Study the drawing (mm; zero at the part's minimum x, y, z) and answer. A direction names the side the tool comes from. Coordinates: 2 decimals unless noted, no trailing zeros. Order: outer loops, then holes, each group sorted by start corner. A loop starts at its lowest first (then second) coordinate and runs counter-clockwise, first axis right, second up. Notation, with made-up numbers: M 7.25,83 L 25.25,83 A36 ccw 25.25,119 Z; hole C 25.25,-2.75 d10. An arc over 180 degrees is marked long. Use a Markdown table: item, result. Add a question column.
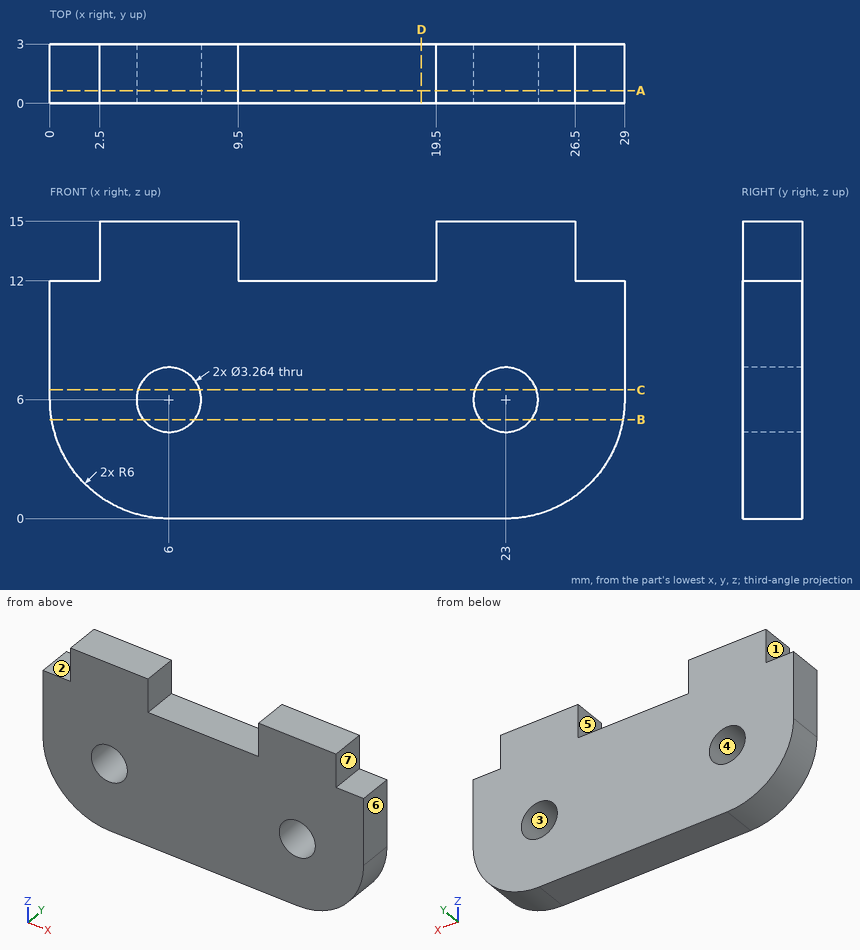
(1) A cutting plane is placed at B-B on z = 5. Write down the section's boundary in (x, y).
(2) The mould has two halves that part along X. Classify the marked faces 1, 2, 3 and 4: pulls with the +X half, pulls with the -X half, needs draft (parallel to the pull), parting line crosses it, or undercut.
(3) A cutting plane is placed at D-D on x = 18.75. Write down the section's boundary in (y, z).
(4) Straight lines are drawn through the part: line 1 (X direction, y = 2.2, z = 6); line 2 (Z direction, x = 23, y = 0.7); line 3 (X direction, y = 2.6, z = 6.75). For each, find the intervals that lie inside material, in ascending order.
(5) A cutting plane is placed at C-C on z = 6.5. Write down the section's boundary in (x, y).
(6) Given P1, Ø1, axis at x = 7.5, y = 2, coming from the -Z side; P2, Ø1.2, axis at x = 27.5, y = 1, coming from the +Z side; P3, Ø1.5, axis at x = 3, y = 2.5, coming from the -Z side; P4, Ø1.5, axis at y = 2, z = 13, coming from the +X side, each flat-ended and moving along its own axis, determine where each tip first touches the part or whether it passes through.
(7) Which of the six approach directions +Z, -Z, +X, -X, +Y, -Y give full straight-line access (tool end or side, diameter ignored) to the marked faces 5, 6 and 7?
(8) A cutting plane is placed at A-A on y = 0.65. Write down the section's boundary in (x, z).
From the geometry:
| question | item | result |
|---|---|---|
| 1 | outline | M 0.08,0 L 4.71,0 L 4.71,3 L 0.08,3 Z; M 7.29,0 L 21.71,0 L 21.71,3 L 7.29,3 Z; M 24.29,0 L 28.92,0 L 28.92,3 L 24.29,3 Z |
| 2 | face 1 | pulls with the -X half |
| 2 | face 2 | needs draft |
| 2 | face 3 | undercut |
| 2 | face 4 | undercut |
| 3 | outline | M 0,0 L 3,0 L 3,12 L 0,12 Z |
| 4 | line 1 | x = 0 to 4.37, 7.63 to 21.37, 24.63 to 29 |
| 4 | line 2 | z = 0 to 4.37, 7.63 to 15 |
| 4 | line 3 | x = 0 to 4.55, 7.45 to 21.55, 24.45 to 29 |
| 5 | outline | M 0,0 L 4.45,0 L 4.45,3 L 0,3 Z; M 7.55,0 L 21.45,0 L 21.45,3 L 7.55,3 Z; M 24.55,0 L 29,0 L 29,3 L 24.55,3 Z |
| 6 | P1 | stops at z = 0 |
| 6 | P2 | stops at z = 12 |
| 6 | P3 | stops at z = 0.44 |
| 6 | P4 | stops at x = 26.5 |
| 7 | face 5 | +Z, +Y, -Y |
| 7 | face 6 | +Z, -Z, +X, +Y, -Y |
| 7 | face 7 | +Z, +X, +Y, -Y |
| 8 | outline | M 0,6 A6 ccw 6,0 L 23,0 A6 ccw 29,6 L 29,12 L 26.5,12 L 26.5,15 L 19.5,15 L 19.5,12 L 9.5,12 L 9.5,15 L 2.5,15 L 2.5,12 L 0,12 Z; hole C 6,6 d3.26; hole C 23,6 d3.26 |
